Design review of the part built by this model. Coordinates are the model's own, in mm. Face numbers are marked on the shaded views. A direction names the side the tool comes from. Give positions to 0.01 mm unless a question says otherwise; leave off trailing zeros. Loops run counter-clockwise (first coordinate to the right, second up) from the corner with the lowest first, then second, coordinate; pieces in that order, holes last.
Autodesk Fusion 360 part; units mm, degrees
sketch "Sketch1" plane through (0, 0, 0) normal (0, 1, 0) x (1, 0, 0)
  line L0 (-4.7, 2.7) -> (4.7, 2.7)
  line L1 (4.7, 2.7) -> (4.7, -2.7)
  line L2 (4.7, -2.7) -> (-4.7, -2.7)
  line L3 (-4.7, -2.7) -> (-4.7, 2.7)
  line L4 (-4.7, 2.7) -> (4.7, -2.7) construction
  line L5 (4.7, 2.7) -> (-4.7, -2.7) construction
  line L6 (-5.7, 3.7) -> (5.7, 3.7)
  line L7 (5.7, 3.7) -> (5.7, -3.7)
  line L8 (5.7, -3.7) -> (-5.7, -3.7)
  line L9 (-5.7, -3.7) -> (-5.7, 3.7)
  circle A0 centre (5.7, 3.7) radius 4
  line L10 (-4.7, 2.7) -> (-5.7, 2.7)
  dimension "d1" = 9.4
  dimension "d2" = 5.4
  dimension "d3" = -1
  dimension "d12" = 8
extrude "Extrude1" add sketch "Sketch1" along normal blind 4 contours L0 L6 L9 A0 L10 | L1 L2 L3 L7 L8 L9 A0 L10 | L0 L1 L6 L7 A0
extrude "Extrude2" add sketch "Sketch1" along normal blind 1 contours L0 L1 L2 L3 A0 | L0 L1 A0
sketch "Sketch2" plane through (0, 0, 0) normal (0, 1, 0) x (1, 0, 0)
  line L0 (-5.7, -3.7) -> (5.7, -3.7)
  line L1 (5.7, -3.7) -> (5.7, -2.7)
  line L2 (5.7, -2.7) -> (-5.7, -2.7)
  line L3 (-5.7, -2.7) -> (-5.7, -3.7)
  point P0 (-5.7, -3.7)
  dimension "d8" = 1
  dimension "d11" = 11.4
extrude "Extrude3" add sketch "Sketch2" against normal blind 2
extrude "Extrude4" cut sketch "Sketch1" along normal blind 5 contours L0 L1 L6 L7 A0 | L0 L1 A0
extrude "Extrude5" add sketch "Sketch1" along normal blind 5.5 contours L0 L6 L9 A0 L10
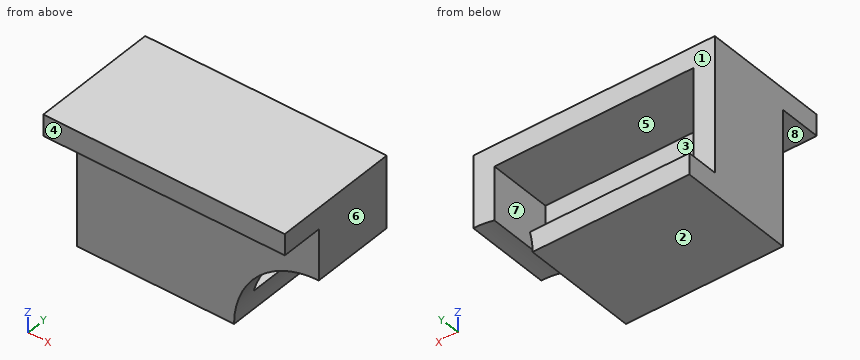
Q1. Draft analysis for pull direction Z (two halves, no side actions). For the marked faces 1, 2 and 3, state which applies: pulls with the +Z half, pulls with the -Z half, needs draft (parallel to the pull), parting line crosses it, or undercut.
Results:
face 1: needs draft
face 2: pulls with the -Z half
face 3: undercut
Q2. Take a section at B-B (x = 4). Give the boundary of the cut face in (y, z).
Results:
outline: (-2, 2.7) - (0, 2.7) - (0, -0.08) - (1, -0.08) - (1, 2.7) - (4, 2.7) - (4, 3.7) - (-2, 3.7) - close
Q3. Take a section at C-C (y = 2). Give the boundary of the cut face in (x, z), plus the area to 3 significant figures.
Results:
outline: (-5.7, -3.7) - (1.7, -3.7) arc R4 cw to (1.83, -2.7) - (-4.7, -2.7) - (-4.7, 2.7) - (4.7, 2.7) - (4.7, 0.17) arc R4 cw to (5.7, 0.3) - (5.7, 3.7) - (-5.7, 3.7) - close
area: 26.7 mm2
Q4. Insertion check: pin 1 (1.9 mm diameter, centred on x = -2.5, z = -0.5, fed in from -Y); pin 2 (1.6 mm diameter, centred on x = 0.5, z = -0.5, fed in from +Y); pin 3 (1.6 mm diameter, centred on x = 1, y = -1, fed in from -Z). Each pin has a flat end and moves straight along its axis. Give the tip position at first contact, or say it passes through.
Results:
pin 1: stops at y = 0
pin 2: stops at y = 1
pin 3: stops at z = 2.7
Q5. Take a section at D-D (x = -3.75). Give the boundary of the cut face in (y, z).
Results:
outline: (-2, 2.7) - (0, 2.7) - (0, -3.7) - (5.5, -3.7) - (5.5, -2.7) - (1, -2.7) - (1, 2.7) - (4, 2.7) - (4, 3.7) - (-2, 3.7) - close
Q6. Take a section at A-A (z = 1.5). Give the boundary of the cut face in (x, y), plus the area to 3 significant figures.
Results:
outline: (-5.7, 0) - (5.7, 0) - (5.7, 4) - (4.7, 4) - (4.7, 1) - (-4.7, 1) - (-4.7, 4) - (-5.7, 4) - close
area: 17.4 mm2
Q7. Tool access review of the marked faces 4, 5, 6, 7 and 8: name each direction out of +Z, -Z, +X, -X, +Y, -Y from which nothing blocks a thin tool from reaching the whole face with its end or side.
Results:
face 4: +Z, -Z, +X, -X, -Y
face 5: +Y
face 6: +Z, -Z, +X, +Y, -Y
face 7: -Z, +Y
face 8: -Z, +X, -X, -Y
Q8. Wall thickness on line 1 (Z direction, x = 0.5, y = 3); line 2 (Y direction, x = -4.5, z = 1.75); line 3 (Z direction, x = 0.75, y = 5): over which ranges is each line inside the solid? List them lowest first.
Results:
line 1: z = -3.7 to -2.7, 2.7 to 3.7
line 2: y = 0 to 1
line 3: z = -3.7 to -2.7
